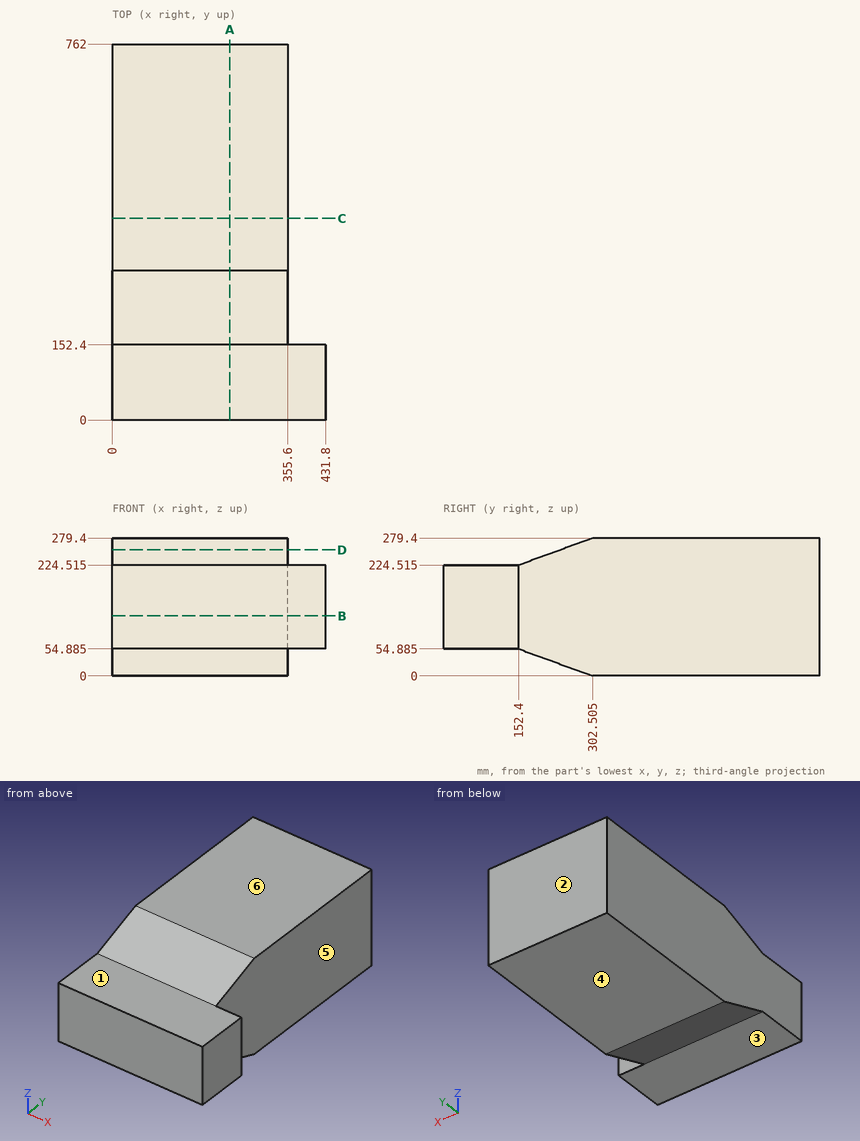
Geometry check sheet. Reference: drawing and pictorial views, mm from the part's lowest x, y, z. A direction names the side the tool comes from. Round coordinates to 2 decimals unless told otherwise and drop trailing zeros. Loops run counter-clockwise (first coordinate to the right, second up) from the corner with the lowest first, then second, coordinate; pieces in that order, holes last. Notation, with made-up numbers: M -15,73 L 42,73 A35 cw 42,105 Z; hole C -2.75,46 d6. An arc over 180 degrees is marked long. Return JSON: item names as keys, results as strings. Group by question number.
(1) Section check C-C, the plane y = 408.5. Enter the section's corners in (x, z).
(2) Set-up check for the marked faces 1, 2 and 3: record each of +Z, -Z, +X, -X, +Y, -Y from which the full face is reachable in a straight line by a thin tool's end or side.
(3) Section check B-B, the plane z = 122. Enter the section's corners in (x, y), and give its area (3 significant figures).
(4) Mould release check, pull along Z, two halves, no side actions. Record for the marked faces 4, 5 and 6: pulls with the +Z half, pulls with the -Z half, needs draft (parallel to the pull), parting line crosses it, or undercut.
(5) Section check A-A, the plane x = 238. Enter the section's corners in (y, z) (1 decimal).
(6) Scan lines: line 1 along X through (y, z) = (345.5, 255); line 2 along Z through (x, y) = (131.5, 68) (1 decimal); line 3 along Y through (x, z) = (387, 220.5). Record each from-to range of solid material in increasing order. Write a range as [from, to].
(7) Go/stop test with flat-tipped pins: pin 1 (10 mm diameter, centred on y = 223.5, z = 63.5, fed in from +X); pin 2 (2 mm diameter, centred on x = 377.5, z = 106, fed in from +Y). Record where each tip stops, or that it passes through.
(8) Section check D-D, the plane z = 255.5. Enter the section's corners in (x, y), and give its area (3 significant figures).
Data:
{
 "1": {"outline": "M 0,0 L 355.6,0 L 355.6,279.4 L 0,279.4 Z"},
 "2": {"face 1": "+Z, +X, -X, -Y", "face 2": "+Z, -Z, +X, -X, +Y", "face 3": "-Z, +X, -X, -Y"},
 "3": {"outline": "M 0,0 L 431.8,0 L 431.8,152.4 L 355.6,152.4 L 355.6,762 L 0,762 Z", "area": "283,000 mm²"},
 "4": {"face 4": "pulls with the -Z half", "face 5": "needs draft", "face 6": "pulls with the +Z half"},
 "5": {"outline": "M 0,54.9 L 152.4,54.9 L 302.5,0 L 762,0 L 762,279.4 L 302.5,279.4 L 152.4,224.5 L 0,224.5 Z"},
 "6": {"line 1": "[0, 355.6]", "line 2": "[54.9, 224.5]", "line 3": "[0, 152.4]"},
 "7": {"pin 1": "x = 355.6", "pin 2": "y = 152.4"},
 "8": {"outline": "M 0,237.14 L 355.6,237.14 L 355.6,762 L 0,762 Z", "area": "187,000 mm²"}
}
